Source: CAD feature listing. Evaluate the final solid. Frame: model axes, mm. Face numbers are marked on the shaded views. A direction names the side the tool comes from. Give positions to 0.01 mm unless a question says otherwise; leave off trailing zeros. Order: outer loops, then holes, each group sorted by start corner. A loop starts at its lowest first (then second) coordinate and runs counter-clockwise, first axis right, second up.
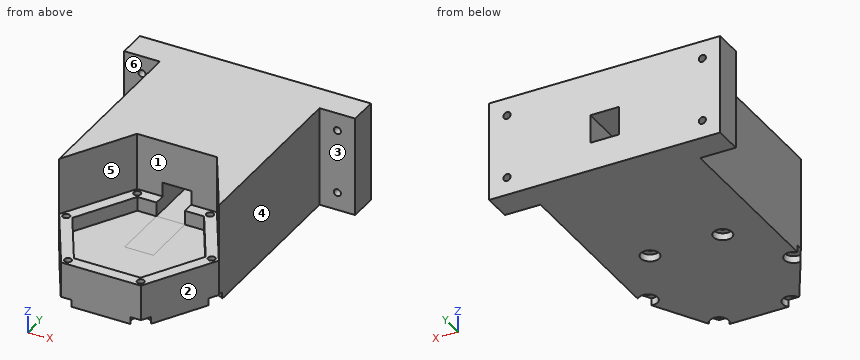
Autodesk Inventor part; units mm, degrees
ref_plane "YZ Plane" through (0, 0, 0) normal (1, 0, 0) x (0, 1, 0)
ref_plane "XZ Plane" through (0, 0, 0) normal (0, 1, 0) x (-1, 0, 0)
ref_plane "XY Plane" through (0, 0, 0) normal (0, 0, 1) x (1, 0, 0)
sketch "Sketch5" plane through (0, 0, 0) normal (0, 0, 1) x (1, 0, 0)
  line L0 (56, 0) -> (28, -48.4974)
  line L1 (28, -48.4974) -> (-28, -48.4974)
  line L2 (-28, -48.4974) -> (-56, 0)
  line L3 (-56, 0) -> (-28, 48.4974)
  line L4 (-28, 48.4974) -> (28, 48.4974)
  line L5 (28, 48.4974) -> (56, 0)
  circle A0 centre (0, 30) radius 2.5
  circle A1 centre (-25.9808, 15) radius 2.5
  circle A2 centre (-25.9808, -15) radius 2.5
  circle A3 centre (0, -30) radius 2.5
  circle A4 centre (25.9808, -15) radius 2.5
  circle A5 centre (25.9808, 15) radius 2.5
  point P0 (0, 0)
  point P1 (0, 0)
  dimension "d28" = 112
  dimension "d29" = 5
  dimension "d30" = 30
  dimension "d33" = 360
extrude "Extrusion3" add sketch "Sketch5" along normal blind 10
sketch "Sketch6" plane through (0, 0, 10) normal (0, 0, 1) x (1, 0, 0)
  circle A0 centre (25.9808, 15) radius 2.5 construction
  circle A1 centre (25.9808, -15) radius 2.5 construction
  circle A2 centre (0, -30) radius 2.5 construction
  circle A3 centre (-25.9808, -15) radius 2.5 construction
  circle A4 centre (-25.9808, 15) radius 2.5 construction
  circle A5 centre (0, 30) radius 2.5 construction
  line L0 (28, -48.4974) -> (56, 0)
  line L1 (56, 0) -> (28, 48.4974)
  line L2 (28, 48.4974) -> (-28, 48.4974)
  line L3 (-28, 48.4974) -> (-56, 0)
  line L4 (-56, 0) -> (-28, -48.4974)
  line L5 (-28, -48.4974) -> (28, -48.4974)
  line L6 (-44.453, 0) -> (-22.2265, 38.4974)
  line L7 (-22.2265, 38.4974) -> (22.2265, 38.4974)
  line L8 (22.2265, 38.4974) -> (44.453, 0)
  line L9 (44.453, 0) -> (22.2265, -38.4974)
  line L10 (22.2265, -38.4974) -> (-22.2265, -38.4974)
  line L11 (-22.2265, -38.4974) -> (-44.453, 0)
  point P0 (0, 0)
  dimension "d37" = 10
extrude "Extrusion4" add sketch "Sketch6" along normal blind 50
sketch "Sketch7" plane through (0, 0, 60) normal (0, 0, 1) x (1, 0, 0)
  line L0 (-22.2265, 38.4974) -> (22.2265, 38.4974)
  line L1 (22.2265, 38.4974) -> (44.453, 0)
  line L2 (44.453, 0) -> (22.2265, -38.4974)
  line L3 (22.2265, -38.4974) -> (-22.2265, -38.4974)
  line L4 (-22.2265, -38.4974) -> (-44.453, 0)
  line L5 (-44.453, 0) -> (-22.2265, 38.4974)
  line L6 (28, -48.4974) -> (56, 0)
  line L7 (56, 0) -> (28, 48.4974)
  line L8 (28, 48.4974) -> (-28, 48.4974)
  line L9 (-28, 48.4974) -> (-56, 0)
  line L10 (-56, 0) -> (-28, -48.4974)
  line L11 (-28, -48.4974) -> (28, -48.4974)
  point P0 (0, 0)
extrude "Extrusion5" add sketch "Sketch7" along normal blind 10 contours L0 L1 L2 L3 L4 L5 | L11 L10 L9 L8 L7 L6
sketch "Sketch8" plane through (-28, 48.4974, 0) normal (0, 1, 0) x (1, 0, 0)
  line L0 (-28, -70) -> (0, -70)
  line L1 (-28, -70) -> (84, -70)
  line L2 (84, -70) -> (84, 0)
  line L3 (84, 0) -> (-28, 0)
  line L4 (-28, 0) -> (-28, -70)
  line L5 (0, 0) -> (56, 0)
  point P0 (28, 0)
  point P1 (28, 0)
  dimension "d42" = 112
extrude "Extrusion6" add sketch "Sketch8" against normal blind 48.4974 and the other way blind 100
sketch "Sketch9" plane through (-28, 148.4974, 0) normal (0, 1, 0) x (1, 0, 0)
  line L0 (-16.453, -60) -> (72.453, -60)
  line L1 (72.453, -10) -> (72.453, -60)
  line L2 (-16.453, -10) -> (-16.453, -60)
  line L3 (50.2265, -10) -> (72.453, -10)
  line L4 (72.453, -10) -> (-16.453, -10)
  point P0 (28, 0)
extrude "Extrusion7" cut sketch "Sketch9" against normal blind 100
sketch "Sketch10" plane through (0, 0, 0) normal (0, 0, -1) x (-1, 0, 0)
  circle A0 centre (-25.9808, -15) radius 2.5
  circle A1 centre (-25.9808, -15) radius 2.5
  circle A2 centre (-25.9808, -15) radius 2.5
  circle A3 centre (0, -30) radius 2.5
  circle A4 centre (25.9808, -15) radius 2.5
  circle A5 centre (25.9808, 15) radius 2.5
  circle A6 centre (0, 30) radius 2.5
  circle A7 centre (-25.9808, 15) radius 2.5
  point P0 (0, 0)
  dimension "d52" = 360
extrude "Extrusion8" cut sketch "Sketch10" against normal blind 10
sketch "Sketch12" plane through (0, 0, 70) normal (0, 0, 1) x (1, 0, 0)
  line L0 (56, 0) -> (28, -48.4974)
  line L1 (56, 0) -> (28, -48.4974)
  line L2 (28, -48.4974) -> (-28, -48.4974)
  line L3 (-28, -48.4974) -> (-56, 0)
  line L4 (-56, 0) -> (-28, 48.4974)
  line L5 (-28, 48.4974) -> (28, 48.4974)
  line L6 (28, 48.4974) -> (56, 0)
  point P0 (0, 0)
  point P1 (0, 0)
extrude "Extrusion9" cut sketch "Sketch12" against normal blind 50
sketch "Sketch13" plane through (0, 0, 10) normal (0, 0, 1) x (1, 0, 0)
  line L0 (22.2265, -38.4974) -> (44.453, 0)
  line L1 (22.2265, -38.4974) -> (-22.2265, -38.4974)
  line L2 (-22.2265, -38.4974) -> (-44.453, 0)
  line L3 (-44.453, 0) -> (-22.2265, 38.4974)
  line L4 (-22.2265, 38.4974) -> (22.2265, 38.4974)
  line L5 (22.2265, 38.4974) -> (44.453, 0)
  line L6 (44.453, 0) -> (22.2265, -38.4974)
  point P0 (0, 0)
  point P1 (0, 0)
extrude "Extrusion10" cut sketch "Sketch13" along normal blind 10
sketch "Sketch14" plane through (-44.453, 148.4974, 10) normal (0, 0, 1) x (1, 0, 0)
  line L0 (-11.547, -148.4974) -> (16.453, -100)
  line L1 (16.453, -100) -> (16.453, -120)
  line L2 (0, -148.4974) -> (22.2265, -110)
  line L3 (16.453, -100) -> (72.453, -100)
  line L4 (72.453, -100) -> (72.453, -120)
  line L5 (66.6795, -110) -> (88.906, -148.4974)
  line L6 (16.453, -120) -> (72.453, -120)
  line L7 (16.453, -100) -> (72.453, -100)
  point P0 (44.453, -148.4974)
extrude "Extrusion11" cut sketch "Sketch14" along normal blind 10
sketch "Sketch15" plane through (-28, 148.4974, 0) normal (0, 1, 0) x (1, 0, 0)
  line L0 (-28, -20) -> (-28, -70)
  line L1 (-28, -70) -> (-53, -70)
  line L2 (-53, -70) -> (-53, 0)
  line L3 (-53, 0) -> (-28, 0)
  line L4 (-28, 0) -> (-28, -70)
  line L5 (-28, -70) -> (84, -70)
  line L6 (84, -70) -> (109, -70)
  line L7 (109, -70) -> (109, 0)
  line L8 (109, 0) -> (84, 0)
  line L9 (84, 0) -> (84, -70)
  circle A0 centre (96.5, -57.5) radius 2.5
  circle A1 centre (96.5, -12.5) radius 2.5
  circle A2 centre (-40.5, -12.5) radius 2.5
  circle A3 centre (-40.5, -57.5) radius 2.5
  line L10 (96.5, -57.5) -> (96.5, -12.5) construction
  line L11 (-40.5, -12.5) -> (-40.5, -57.5) construction
  point P0 (28, 0)
  point P1 (-40.5, -70)
  point P2 (-40.5, 0)
  point P3 (96.5, 0)
  point P4 (96.5, -70)
  point P5 (96.5, -35)
  point P6 (109, -35)
  dimension "d62" = 25
  dimension "d63" = 25
  dimension "d64" = 5
  dimension "d65" = 5
  dimension "d66" = 5
  dimension "d67" = 5
  dimension "d68" = 45
extrude "Extrusion12" add sketch "Sketch15" against normal blind 20
sketch "Sketch16" plane through (-28, 48.4974, 0) normal (0, 1, 0) x (1, 0, 0)
  line L0 (0, -20) -> (0, -10)
  line L1 (-16.453, -10) -> (0, -10)
  line L2 (-16.453, -60) -> (-16.453, -10)
  line L3 (0, -60) -> (-16.453, -60)
  line L4 (0, -60) -> (0, -20)
  line L5 (72.453, -10) -> (72.453, -60)
  line L6 (56, -10) -> (56, -20)
  line L7 (56, -20) -> (56, -60)
  line L8 (72.453, -60) -> (56, -60)
  line L9 (72.453, -10) -> (72.453, -60)
  line L10 (56, -10) -> (72.453, -10)
  point P0 (28, 0)
extrude "Extrusion13" add sketch "Sketch16" along normal blind 100
sketch "Sketch17" plane through (0, 0, 0) normal (0, 0, -1) x (-1, 0, 0)
  circle A0 centre (-51, 0) radius 2.5
  circle A1 centre (-25.5, -44.1673) radius 2.5
  circle A2 centre (25.5, -44.1673) radius 2.5
  circle A3 centre (51, 0) radius 2.5
  circle A4 centre (25.5, 44.1673) radius 2.5
  circle A5 centre (-25.5, 44.1673) radius 2.5
  point P0 (0, 0)
  point P1 (-56, 0)
  dimension "d73" = 5
  dimension "d74" = 5
  dimension "d77" = 360
extrude "Extrusion14" cut sketch "Sketch17" against normal through all
sketch "Sketch18" plane through (0, 0, 0) normal (0, 0, -1) x (-1, 0, 0)
  circle A0 centre (-51, 0) radius 2.5
  circle A1 centre (-51, 0) radius 6.5
  circle A2 centre (-25.5, 44.1673) radius 6.5
  circle A3 centre (25.5, 44.1673) radius 6.5
  circle A4 centre (51, 0) radius 6.5
  circle A5 centre (25.5, -44.1673) radius 6.5
  circle A6 centre (-25.5, -44.1673) radius 6.5
  point P0 (0, 0)
  dimension "d81" = 13
  dimension "d84" = 360
extrude "Extrusion15" cut sketch "Sketch18" against normal blind 5 contours A0 | A1 | A2 | A3 | A4 | A5 | A6
sketch "Sketch19" plane through (0, 0, 10) normal (0, 0, 1) x (1, 0, 0)
  circle A0 centre (0, -30) radius 2.5
  circle A1 centre (-25.9808, -15) radius 2.5
  circle A2 centre (-25.9808, 15) radius 2.5
  circle A3 centre (0, 30) radius 2.5
  circle A4 centre (25.9808, 15) radius 2.5
  circle A5 centre (25.9808, -15) radius 2.5
  point P0 (0, 0)
extrude "Extrusion16" add sketch "Sketch19" against normal blind 10
sketch "Sketch20" plane through (-28, 148.4974, 0) normal (0, 1, 0) x (1, 0, 0)
  line L0 (56, -60) -> (0, -60)
  line L1 (0, -60) -> (0, -10)
  line L2 (0, -10) -> (56, -10)
  line L3 (56, -10) -> (56, -60)
  line L4 (5.7735, -20) -> (50.2265, -20)
  line L5 (50.2265, -20) -> (72.453, -20)
  line L6 (-16.453, -20) -> (5.7735, -20)
  line L7 (56, -20) -> (56, -10)
  line L8 (56, -20) -> (0, -20)
  line L9 (0, -20) -> (0, -60)
  line L10 (0, -60) -> (56, -60)
  line L11 (56, -60) -> (56, -20)
  point P0 (28, 0)
extrude "Extrusion17" add sketch "Sketch20" against normal blind 100 contours L0 L1 L6 L4 L5 L3
sketch "Sketch21" plane through (0, 0, 10) normal (0, 0, 1) x (1, 0, 0)
  line L0 (-28, 148.4974) -> (-28, 44.1673)
  circle A0 centre (-25.5, 44.1673) radius 2.5
  line L1 (-28, 44.1673) -> (-28, 28.4974)
  line L2 (-44.453, 0) -> (-28, 28.4974)
  line L3 (-44.453, 0) -> (-22.2265, -38.4974)
  line L4 (-22.2265, -38.4974) -> (22.2265, -38.4974)
  line L5 (22.2265, -38.4974) -> (44.453, 0)
  line L6 (28, 28.4974) -> (44.453, 0)
  line L7 (28, 28.4974) -> (28, 44.1673)
  circle A1 centre (25.5, 44.1673) radius 2.5
  line L8 (28, 44.1673) -> (28, 148.4974)
  line L9 (-28, 148.4974) -> (28, 148.4974)
  point P0 (0, 0)
extrude "Extrusion18" add sketch "Sketch21" along normal blind 10
sketch "Sketch22" plane through (0, 0, 20) normal (0, 0, 1) x (1, 0, 0)
  circle A0 centre (25.5, 44.1673) radius 2.5
  line L0 (-28, 48.4974) -> (28, 48.4974)
  line L1 (-56, 0) -> (-28, 48.4974)
  line L2 (-28, -48.4974) -> (-56, 0)
  line L3 (28, -48.4974) -> (-28, -48.4974)
  line L4 (56, 0) -> (28, -48.4974)
  line L5 (28, 48.4974) -> (56, 0)
  circle A1 centre (-25.5, -44.1673) radius 2.5
  circle A2 centre (51, 0) radius 2.5
  circle A3 centre (25.5, -44.1673) radius 2.5
  circle A4 centre (-51, 0) radius 2.5
  circle A5 centre (-25.5, 44.1673) radius 2.5
  line L6 (-46.7624, 0) -> (-23.3812, 40.4974)
  line L7 (-23.3812, 40.4974) -> (23.3812, 40.4974)
  line L8 (23.3812, 40.4974) -> (46.7624, 0)
  line L9 (46.7624, 0) -> (23.3812, -40.4974)
  line L10 (23.3812, -40.4974) -> (-23.3812, -40.4974)
  line L11 (-23.3812, -40.4974) -> (-46.7624, 0)
  point P0 (0, 0)
  dimension "d94" = 8
extrude "Extrusion19" add sketch "Sketch22" along normal blind 10
sketch "Sketch23" plane through (0, 0, 20) normal (0, 0, 1) x (1, 0, 0)
  line L0 (-10, 0) -> (10, 0)
  line L1 (10, 0) -> (10, 148.4974)
  line L2 (10, 148.4974) -> (-10, 148.4974)
  line L3 (-10, 148.4974) -> (-10, 0)
  line L4 (-81, 148.4974) -> (81, 148.4974)
  point P0 (0, 0)
  point P1 (0, 0)
  point P2 (0, 148.4974)
  dimension "d97" = 20
extrude "Extrusion20" cut sketch "Sketch23" along normal blind 20
properties part number "TARM01" material "ABS Plastic"
1) Section query A-A, the plane x = 68.5. Return the cut outline in (y, z).
Report:
outline: (128.5, 0) - (148.5, 0) - (148.5, 10) - (128.5, 10) - close; (128.5, 15) - (148.5, 15) - (148.5, 55) - (128.5, 55) - close; (128.5, 60) - (148.5, 60) - (148.5, 70) - (128.5, 70) - close
2) Draft query along X for the marked faces 1, 2 and 3. Return one class per face: +X half, -X half, draft (parallel to the pull), parting line (faces both ways), or undercut.
Report:
face 1: undercut
face 2: +X half
face 3: draft
3) Pin query (flat end, axial travel): pin 1 (1 mm diameter, centred on y = 53, z = 50.5, fed in from -X); pin 2 (10 mm diameter, centred on x = -0.5, y = 21.5, fed in from +Z); pin 3 (6 mm diameter, centred on x = 6.5, z = 44.5, fed in from -Y). Return the tip coordinate at first contact, or that it passes through.
Report:
pin 1: stops at x = -56
pin 2: stops at z = 20
pin 3: stops at y = 48.5
4) Section query B-B, the plane z = 37. Return the cut outline in (x, y).
Report:
outline: (-81, 128.5) - (-56, 128.5) - (-56, 0) - (-28, 48.5) - (-10, 48.5) - (-10, 148.5) - (-81, 148.5) - close; (10, 48.5) - (28, 48.5) - (56, 0) - (56, 128.5) - (81, 128.5) - (81, 148.5) - (10, 148.5) - close
5) Section query D-D, the plane z = 12.5. Count the separate pieces of the cut face and the enclosed holes in it, and give its area (3 significant figures).
Report:
separate pieces: 3
enclosed holes: 6
area: 21,400 mm2
6) Section query C-C, the plane y = 62. Return the cut outline in (x, z).
Report:
outline: (-56, 0) - (56, 0) - (56, 70) - (-56, 70) - close; hole (-10, 20) - (10, 20) - (10, 40) - (-10, 40) - close
7) Reachability of the marked faces 4, 5 and 6 from +Z, -Z, +X, -X, +Y, -Y: full face, straight path, thin tool, end or side. Return the list, or none.
Report:
face 4: +Z, -Z, +X, -Y
face 5: +Z, -Y
face 6: +Z, -Z, -X, -Y
8) Material intervals for L1, parallel to Y at x = 25.5, z = 15; L2, parallel to Y at x = -25, z = 8; L3, parallel to X at y = 143, z = 57.5, sorted ascending.
Report:
L1: y = -48.5 to -46.67, -41.67 to 41.67, 46.67 to 148.5
L2: y = -48.5 to -46.62, -41.72 to 41.72, 46.62 to 148.5
L3: x = -81 to -71, -66 to 66, 71 to 81
